from build123d import *

# Parameters (mm, degrees)
EXTRUDE_1_DEPTH          = 245
CUT_EXTRUDE_1_DEPTH      = 246.916652547
CUT_EXTRUDE_1_DEPTH_BACK = 246.916652547
SKETCH_2_R               = 2


with BuildPart() as part:
    # 草图1 → 凸台-拉伸1 (new, symmetric)
    with BuildSketch(Plane(origin=(0, 0, 0), x_dir=(1, 0, 0), z_dir=(0, 1, 0))):
        with BuildLine():
            Line((-11, -15), (11, -15))
            ThreePointArc((11, -15), (13.828427125, -13.828427125), (15, -11))
            Line((15, -11), (15, 11))
            ThreePointArc((15, 11), (13.828427125, 13.828427125), (11, 15))
            Line((11, 15), (-11, 15))
            ThreePointArc((-11, 15), (-13.828427125, 13.828427125), (-15, 11))
            Line((-15, 11), (-15, -11))
            ThreePointArc((-15, -11), (-13.828427125, -13.828427125), (-11, -15))
        make_face()
        with BuildLine():
            Line((-11, -13), (11, -13))
            ThreePointArc((11, -13), (12.414213562, -12.414213562), (13, -11))
            Line((13, -11), (13, 11))
            ThreePointArc((13, 11), (12.414213562, 12.414213562), (11, 13))
            Line((11, 13), (-11, 13))
            ThreePointArc((-11, 13), (-12.414213562, 12.414213562), (-13, 11))
            Line((-13, 11), (-13, -11))
            ThreePointArc((-13, -11), (-12.414213562, -12.414213562), (-11, -13))
        make_face(mode=Mode.SUBTRACT)
    extrude(amount=EXTRUDE_1_DEPTH, both=True)

    # 草图2 → 切除-拉伸1 (cut, two sides: drawn at the far end of the back side and taken through both)
    with BuildSketch(Plane.XY.offset(-CUT_EXTRUDE_1_DEPTH_BACK)):
        with Locations((0, 55)):
            Circle(SKETCH_2_R)
        with Locations((0, -55)):
            Circle(SKETCH_2_R)
    extrude(amount=CUT_EXTRUDE_1_DEPTH + CUT_EXTRUDE_1_DEPTH_BACK, mode=Mode.SUBTRACT)


solid = part.part
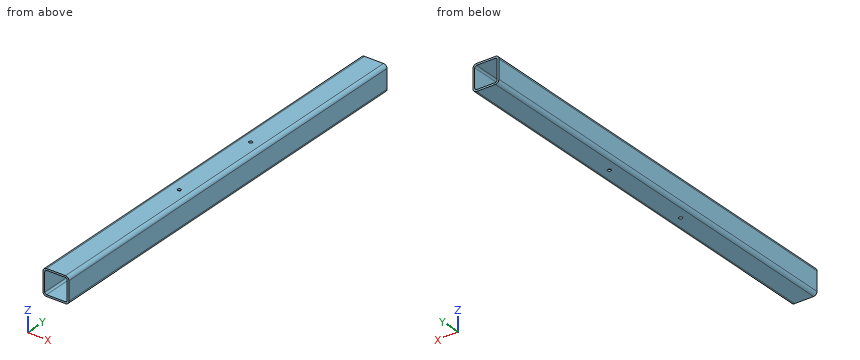
Can you work these out from the model? Positions are in its coordinate system, mm. Give positions to 0.01 mm unless a question says otherwise; leave off trailing zeros. Loops run counter-clockwise (first coordinate to the right, second up) from the corner with the lowest first, then second, coordinate; pieces in that order, holes last. Notation, with made-up numbers: M 78.25,-16 L 104.25,-16 A9 cw 104.25,-1 Z; hole C 64,59 d3. An arc over 180 degrees is marked long. One line per item, written item: value. Start each with the question number.
1) If we section it at A-A, the plane x = -7: Write out the boundary of the cut face in (y, z).
2) If I drill on line 1 (Y direction, x = 0, z = 13.8); line 2 (Z direction, x = 0.5, y = 38), over which ranges is the centre line in solid material (lowest first)? Write a range as [from, to].
3) If we section it at C-C, the plane y = -186: Write out the boundary of the cut face in (x, z).
4) If we section it at B-B, the plane z = 3.75: Write out the boundary of the cut face in (x, y), and give its area (3 significant figures).
5) I'm going to push flat-ended pins straight in: pin 1 (12 mm diameter, centred on x = 3, z = 2.5, fed in from -Y); pin 2 (6.5 mm diameter, centred on x = 0, y = 55, fed in from +Z). Where does each tip first touch, or does it pass through?
Completed:
1. outline: M -245,-15 L 245,-15 L 245,-13 L -245,-13 Z; M -245,13 L 245,13 L 245,15 L -245,15 Z
2. line 1: y = [-245, -57], [-53, 53], [57, 245]
2. line 2: z = [-15, -13], [13, 15]
3. outline: M -15,-11 A4 ccw -11,-15 L 11,-15 A4 ccw 15,-11 L 15,11 A4 ccw 11,15 L -11,15 A4 ccw -15,11 Z; hole M -13,-11 A2 ccw -11,-13 L 11,-13 A2 ccw 13,-11 L 13,11 A2 ccw 11,13 L -11,13 A2 ccw -13,11 Z
4. outline: M -15,-245 L -13,-245 L -13,245 L -15,245 Z; M 13,-245 L 15,-245 L 15,245 L 13,245 Z
4. area: 1,960 mm^2
5. pin 1: passes through
5. pin 2: stops at z = 15
